Work out the finished part from the listing and answer in its coordinate system (mm). Face numbers are marked on the shaded views. A direction names the side the tool comes from. Round coordinates to 2 decimals unless told otherwise and drop trailing zeros. Write each loop counter-clockwise with the first axis right and the second up, starting at its lowest first coordinate (ties: lowest second). Pieces come first, ordered by that corner, then holes. Notation, with made-up numbers: (59, -36) -> (112, -36) arc R29 cw to (112, -4) -> close; hole circle Ø4 at (29.5, 30.5). An arc over 180 degrees is marked (long way). One line per item, written item: value.
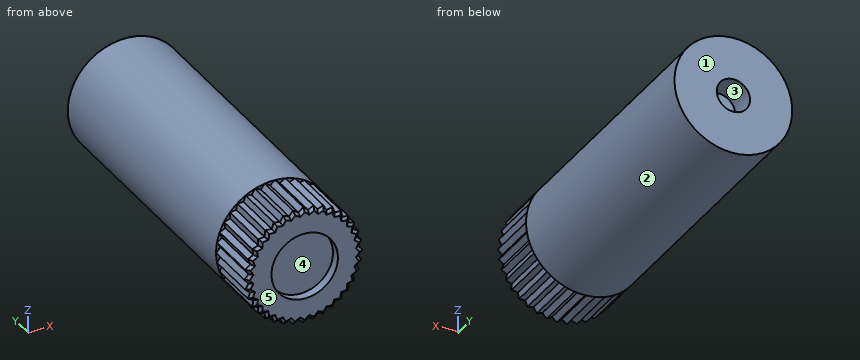
```python
from build123d import *

# Parameters (mm, degrees)
F0_R     = 6.2
F1_DEPTH = 30
F3_DEPTH = 6
F4_SIZE  = 0.3
F5_R     = 3.5
F6_DEPTH = 1
F7_R     = 1.75
F8_DEPTH = 3


with BuildPart() as f1:
    # F0 (on Front) → F1 (new body)
    with BuildSketch(Plane.XZ):
        Circle(F0_R)
    extrude(amount=F1_DEPTH)

    # F2 (on face) → F3 (join)
    with BuildSketch(Plane.XZ.offset(30)):
        Polygon((5.761109, -0.504032), (6.2, 0), (5.761109, 0.504032), (6.105808, 1.076619), (5.586061, 1.496781), (5.826094, 2.120525), (5.241283, 2.44405), (5.369358, 3.1), (4.737251, 3.317059), (4.749476, 3.985283), (4.08928, 4.08928), (3.985283, 4.749476), (3.317059, 4.737251), (3.1, 5.369358), (2.44405, 5.241283), (2.120525, 5.826094), (1.496781, 5.586061), (1.076619, 6.105808), (0.504032, 5.761109), (0, 6.2), (-0.504032, 5.761109), (-1.076619, 6.105808), (-1.496781, 5.586061), (-2.120525, 5.826094), (-2.44405, 5.241283), (-3.1, 5.369358), (-3.317059, 4.737251), (-3.985283, 4.749476), (-4.08928, 4.08928), (-4.749476, 3.985283), (-4.737251, 3.317059), (-5.369358, 3.1), (-5.241283, 2.44405), (-5.826094, 2.120525), (-5.586061, 1.496781), (-6.105808, 1.076619), (-5.761109, 0.504032), (-6.2, 0), (-5.761109, -0.504032), (-6.105808, -1.076619), (-5.586061, -1.496781), (-5.826094, -2.120525), (-5.241283, -2.44405), (-5.369358, -3.1), (-4.737251, -3.317059), (-4.749476, -3.985283), (-4.08928, -4.08928), (-3.985283, -4.749476), (-3.317059, -4.737251), (-3.1, -5.369358), (-2.44405, -5.241283), (-2.120525, -5.826094), (-1.496781, -5.586061), (-1.076619, -6.105808), (-0.504032, -5.761109), (0, -6.2), (0.504032, -5.761109), (1.076619, -6.105808), (1.496781, -5.586061), (2.120525, -5.826094), (2.44405, -5.241283), (3.1, -5.369358), (3.317059, -4.737251), (3.985283, -4.749476), (4.08928, -4.08928), (4.749476, -3.985283), (4.737251, -3.317059), (5.369358, -3.1), (5.241283, -2.44405), (5.826094, -2.120525), (5.586061, -1.496781), (6.105808, -1.076619), align=None)
    extrude(amount=F3_DEPTH)

    # F4
    f4_edges = [f1.edges().sort_by_distance(p)[0] for p in [
        (3.651171, -36, -4.743363),
        (4.037282, -36, -4.419378),
        (4.419378, -36, -4.037282),
        (4.743363, -36, -3.651171),
        (5.053304, -36, -3.208529),
        (5.30532, -36, -2.772025),
        (5.533689, -36, -2.282288),
        (5.706078, -36, -1.808653),
        (5.845934, -36, -1.2867),
        (5.933459, -36, -0.790325),
        (5.980555, -36, -0.252016),
        (5.980555, -36, 0.252016),
        (5.933459, -36, 0.790325),
        (5.845934, -36, 1.2867),
        (5.706078, -36, 1.808653),
        (5.533689, -36, 2.282288),
        (5.30532, -36, 2.772025),
        (5.053304, -36, 3.208529),
        (4.743363, -36, 3.651171),
        (4.419378, -36, 4.037282),
        (4.037282, -36, 4.419378),
        (3.651171, -36, 4.743363),
        (3.208529, -36, 5.053304),
        (2.772025, -36, 5.30532),
        (2.282288, -36, 5.533689),
        (1.808653, -36, 5.706078),
        (1.2867, -36, 5.845934),
        (0.790325, -36, 5.933459),
        (0.252016, -36, 5.980555),
        (-0.252016, -36, 5.980555),
        (-0.790325, -36, 5.933459),
        (-1.2867, -36, 5.845934),
        (-1.808653, -36, 5.706078),
        (-2.282288, -36, 5.533689),
        (-2.772025, -36, 5.30532),
        (-3.208529, -36, 5.053304),
        (-3.651171, -36, 4.743363),
        (-4.037282, -36, 4.419378),
        (-4.419378, -36, 4.037282),
        (-4.743363, -36, 3.651171),
        (-5.053304, -36, 3.208529),
        (-5.30532, -36, 2.772025),
        (-5.533689, -36, 2.282288),
        (-5.706078, -36, 1.808653),
        (-5.845934, -36, 1.2867),
        (-5.933459, -36, 0.790325),
        (-5.980555, -36, 0.252016),
        (-5.980555, -36, -0.252016),
        (-5.933459, -36, -0.790325),
        (-5.845934, -36, -1.2867),
        (-5.706078, -36, -1.808653),
        (-5.533689, -36, -2.282288),
        (-5.30532, -36, -2.772025),
        (-5.053304, -36, -3.208529),
        (-4.743363, -36, -3.651171),
        (-4.419378, -36, -4.037282),
        (-4.037282, -36, -4.419378),
        (-3.651171, -36, -4.743363),
        (-3.208529, -36, -5.053304),
        (-2.772025, -36, -5.30532),
        (-2.282288, -36, -5.533689),
        (-1.808653, -36, -5.706078),
        (-1.2867, -36, -5.845934),
        (-0.790325, -36, -5.933459),
        (-0.252016, -36, -5.980555),
        (0.252016, -36, -5.980555),
        (0.790325, -36, -5.933459),
        (1.2867, -36, -5.845934),
        (1.808653, -36, -5.706078),
        (2.282288, -36, -5.533689),
        (2.772025, -36, -5.30532),
        (3.208529, -36, -5.053304),
    ]]
    chamfer(f4_edges, length=F4_SIZE)

    # F5 (on face) → F6 (cut)
    with BuildSketch(Plane.XZ.offset(36)):
        Circle(F5_R)
    extrude(amount=-F6_DEPTH, mode=Mode.SUBTRACT)

    # F7 (on face) → F8 (cut)
    with BuildSketch(Plane(origin=(0, 0, 0), x_dir=(-1, 0, 0), z_dir=(0, 1, 0))):
        Circle(F7_R)
    extrude(amount=-F8_DEPTH, mode=Mode.SUBTRACT)


solid = f1.part
```
(1) Consider probe 1 along Z at (x, y) = (0, -0.8); probe 2 along Y at (x, z) = (-0.75, 0.5); probe 3 along Y at (x, z) = (3, 1.5). Determine where each line is inside the solid, lowest interval first.
Reported:
probe 1: z = -6.2 to -1.75, 1.75 to 6.2
probe 2: y = -35 to -3
probe 3: y = -35 to 0
(2) Flat-ended cylindrical pins translate along their axes: pin 1 Ø0.5 at (x, z) = (-5.5, -2.5) entering from -Y; pin 2 Ø1 at (y, z) = (-10, -1.5) entering from -X; pin 3 Ø3 at (x, y) = (3, -4.5) entering from -Z. Find the tip coordinate at first contact, or state that the pin passes through.
Reported:
pin 1: stops at y = -35.78
pin 2: stops at x = -6.12
pin 3: stops at z = -6.02
(3) Find section A-A on y = -8. Give the vertices of the cut face in (x, z), plus the area to 3 significant figures.
Reported:
outline: circle Ø12.4 at (0, 0)
area: 121 mm2
(4) A tool of negligible diameter and unlimited length cuts with its end or side. For the marked faces 4 and 5, from which of +Z, -Z, +X, -X, +Y, -Y can it reach the whole face along a straight path? Write none if from no direction.
Reported:
face 4: -Y
face 5: +Z, -Z, +X, -X, -Y
(5) For a pull along X with two mould halves and no side action, classify the marked faces 1, 2 and 3 as pulls with the +X half, pulls with the -X half, needs draft (parallel to the pull), parting line crosses it, or undercut.
Reported:
face 1: needs draft
face 2: parting line crosses it
face 3: undercut
